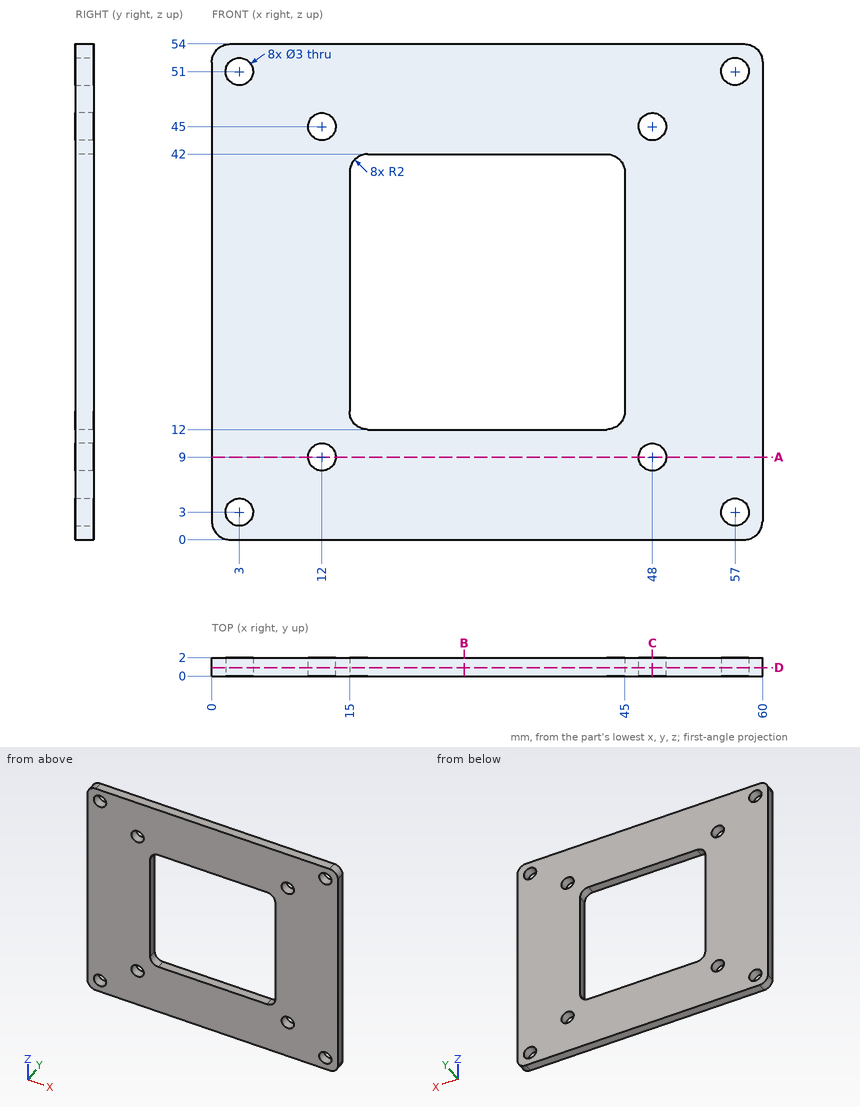
The figure shows three views and two pictorial views of one solid part (mm, origin at its lowest corner). Answer the questions. Round coordinates to 2 decimals unless told otherwise and drop trailing zeros. Loops run counter-clockwise (first coordinate to the right, second up) from the corner with the lowest first, then second, coordinate; pieces in that order, holes last. Notation, with made-up numbers: (-11.75, 51) -> (-1.75, 51) arc R34 ccw to (-1.75, 82) -> close; hole circle Ø5 at (63, -38). An arc over 180 degrees is marked (long way). Use one line per item in the form item = value.
(1) Find section D-D on y = 0.9. Give the number of separate pieces and of enclosed holes in the cut face, then the cut area to 3 significant figures.
Answer list:
separate_pieces = 1
enclosed_holes = 9
area = 2,280 mm2
(2) Find section C-C on x = 48. Give the vertices of the cut face in (y, z).
Answer list:
outline = (0, 0) -> (2, 0) -> (2, 7.5) -> (0, 7.5) -> close; (0, 10.5) -> (2, 10.5) -> (2, 43.5) -> (0, 43.5) -> close; (0, 46.5) -> (2, 46.5) -> (2, 54) -> (0, 54) -> close
(3) Find section B-B on x = 27.5. Give the vertices of the cut face in (y, z).
Answer list:
outline = (0, 0) -> (2, 0) -> (2, 12) -> (0, 12) -> close; (0, 42) -> (2, 42) -> (2, 54) -> (0, 54) -> close
(4) A flat-ended cylindrical pin translates along its axis: P1, Ø5, axis at x = 12, z = 9, coming from the +Y side. Find the tip coordinate at first contact, or state that the pin passes through.
Answer list:
P1 = 2
(5) Straight lines are drawn through the part: line 1 (X direction, y = 0.8, z = 45); line 2 (X direction, y = 1.65, z = 3); line 3 (X direction, y = 1.7, z = 29). For each, find the intervals that lie inside material, in ascending order.
Answer list:
line_1 = 0 to 10.5, 13.5 to 46.5, 49.5 to 60
line_2 = 0 to 1.5, 4.5 to 55.5, 58.5 to 60
line_3 = 0 to 15, 45 to 60
(6) Find section A-A on z = 9. Give the vertices of the cut face in (x, y).
Answer list:
outline = (0, 0) -> (10.5, 0) -> (10.5, 2) -> (0, 2) -> close; (13.5, 0) -> (46.5, 0) -> (46.5, 2) -> (13.5, 2) -> close; (49.5, 0) -> (60, 0) -> (60, 2) -> (49.5, 2) -> close
